The listing builds one solid part. Answer for the finished solid, in the listing's coordinates (mm). Round coordinates to 2 decimals unless told otherwise and drop trailing zeros. Order: outer loops, then holes, each group sorted by start corner. A loop starts at its lowest first (then second) coordinate and runs counter-clockwise, first axis right, second up. Notation, with made-up numbers: (55, 58) - (60, 58) arc R20 ccw to (60, 95) - close; hole circle Ø1 at (72, -4). An arc over 180 degrees is marked (long way). Use CSV: the item, a comma, the result in double quotes. Start each with the question number.
Item 1: Straight lines are drawn through the part: line 1 along X through (y, z) = (-701, -1.85); line 2 along X through (y, z) = (-653, -1.8); line 3 along X through (y, z) = (-699.5, -0.8). For each, find the intervals that lie inside material, in ascending order. Write a range as [from, to].
Item 2: A flat-ended cylindrical pin translates along its axis: P1, Ø9, axis at x = 149.43, y = -806.27, coming from the -Z side. Find the tip coordinate at first contact, or state that the pin passes through.
Item 3: Determine the mould class of faces 1 (the cylindrical face through (12.527, -809.903, -1.232)), 2 (the cylindrical face through (-13, -829.9, -1.2)), 3 (the flat face through (52, -820, -2.5)) for opening direction X: +X half, -X half, draft (parallel to the pull), parting line (faces both ways), or undercut.
Item 4: Find section B-B, the plane z = -0.55. Count the separate pieces of the cut face and the enclosed holes in it, plus the area to 3 significant figures.
Item 5: Find section C-C, the plane y = -788.5. Give the vertices of the cut face in (x, z).
Item 6: Find section A-A, the plane y = -552.5. Give the vertices of the cut face in (x, z), plus the area to 3 significant figures.
```python
from build123d import *

# Parameters (mm, degrees)
BASE_FLANGE1_DEPTH              = 2.5
SKETCH2_W                       = 1968.518691842
SKETCH2_H                       = 782.123286761
CUT_EXTRUDE1_DEPTH              = 10
CUT_EXTRUDE3_DEPTH              = 10
SKETCH10_R                      = 3.5
CUT_EXTRUDE4_DEPTH              = 10
CIRPATTERN1_COUNT               = 10
CIRPATTERN1_ANGLE               = 94.5
CIRPATTERN1_THE_OTHER_WAY_COUNT = 10
CIRPATTERN1_THE_OTHER_WAY_ANGLE = 94.5


# Sheet-metal steps are written as plain solids
with BuildPart() as part:
    # Sketch1 → Base-Flange1 (new body)
    with BuildSketch(Plane.XY):
        with BuildLine():
            Line((829.984939622, -5), (-829.984939622, -5))
            ThreePointArc((-829.984939622, -5), (0, -830), (829.984939622, -5))
        make_face()
    extrude(amount=-BASE_FLANGE1_DEPTH)

    # Sketch2 → Cut-Extrude1 (cut)
    with BuildSketch(Plane.XY):
        with Locations((10.387961435, 27.061643381)):
            Rectangle(SKETCH2_W, SKETCH2_H)
    extrude(amount=-CUT_EXTRUDE1_DEPTH, mode=Mode.SUBTRACT)

    # Sketch9 → Cut-Extrude3 (cut)
    with BuildSketch(Plane.XY):
        with BuildLine():
            Line((-723.60486455, -364), (723.60486455, -364))
            ThreePointArc((723.60486455, -364), (0, -810), (-723.60486455, -364))
        make_face()
    extrude(amount=-CUT_EXTRUDE3_DEPTH, mode=Mode.SUBTRACT)

    # Sketch10 → Cut-Extrude4 (cut)
    with BuildSketch(Plane(origin=(0, 0, -2.5), x_dir=(-1, 0, 0), z_dir=(0, 0, -1))):
        with Locations((0, -820)):
            Circle(SKETCH10_R)
    cut_extrude4 = extrude(amount=-CUT_EXTRUDE4_DEPTH, mode=Mode.SUBTRACT)

    # CirPattern1: Cut-Extrude4 ×10 about axis
    cirpattern1_axis = Axis((0, 0, 0), (0, 0, 1))
    for i in range(1, CIRPATTERN1_COUNT):
        add(cut_extrude4.rotate(cirpattern1_axis, i * CIRPATTERN1_ANGLE / (CIRPATTERN1_COUNT - 1)), mode=Mode.SUBTRACT)

    # CirPattern1 the other way: Cut-Extrude4 ×10 about axis
    cirpattern1_the_other_way_axis = Axis((0, 0, 0), (0, 0, -1))
    for i in range(1, CIRPATTERN1_THE_OTHER_WAY_COUNT):
        add(cut_extrude4.rotate(cirpattern1_the_other_way_axis, i * CIRPATTERN1_THE_OTHER_WAY_ANGLE / (CIRPATTERN1_THE_OTHER_WAY_COUNT - 1)), mode=Mode.SUBTRACT)


solid = part.part
```
Worked out:
1,line 1,"x = [-444.41, -431.43], [-425.47, -405.83], [405.83, 425.47], [431.43, 444.41]"
1,line 2,"x = [-512.34, -479.26], [479.26, 512.34]"
1,line 3,"x = [-446.77, -431.93], [-424.96, -408.41], [408.41, 424.96], [431.93, 446.77]"
2,P1,"stops at z = -2.5"
3,face 1,"undercut"
3,face 2,"parting line"
3,face 3,"draft"
4,separate pieces,"1"
4,enclosed holes,"13"
4,area,"35,900 mm²"
5,outline,"(-259.17, -2.5) - (-185.39, -2.5) - (-185.39, 0) - (-259.17, 0) - close; (185.39, -2.5) - (259.17, -2.5) - (259.17, 0) - (185.39, 0) - close"
6,outline,"(-619.39, -2.5) - (-592.32, -2.5) - (-592.32, 0) - (-619.39, 0) - close; (592.32, -2.5) - (619.39, -2.5) - (619.39, 0) - (592.32, 0) - close"
6,area,"135 mm²"
